Autodesk Inventor part; units mm, degrees
ref_plane "YZ Plane" through (0, 0, 0) normal (1, 0, 0) x (0, 1, 0)
ref_plane "XZ Plane" through (0, 0, 0) normal (0, 1, 0) x (-1, 0, 0)
ref_plane "XY Plane" through (0, 0, 0) normal (0, 0, 1) x (1, 0, 0)
sketch "スケッチ1" plane through (0, 0, 0) normal (1, 0, 0) x (0, 1, 0)
  line L0 (0, 0) -> (30, 0)
  line L1 (30, 0) -> (30, -43)
  line L2 (30, -43) -> (0, -43)
  line L3 (0, -43) -> (0, 0)
  circle A0 centre (15, -5) radius 1.5
  circle A1 centre (15, -38) radius 1.5
  line L4 (30, -21.5) -> (0, -21.5)
  line L5 (30, -18.3) -> (0, -18.3)
  line L6 (30, -24.7) -> (0, -24.7)
  line L7 (15, 0) -> (15, -43)
  line L8 (16.285, -18.3) -> (16.285, -24.7)
  line L9 (13.715, -18.3) -> (13.715, -24.7)
  line L10 (20.08, -18.3) -> (20.08, -24.7)
  line L11 (25.16, -18.3) -> (25.16, -24.7)
  line L12 (30.24, -18.3) -> (30.24, -24.7)
  line L13 (21.365, -18.3) -> (21.365, -24.7)
  line L14 (26.445, -18.3) -> (26.445, -24.7)
  line L15 (28.955, -18.3) -> (28.955, -24.7)
  line L16 (23.875, -18.3) -> (23.875, -24.7)
  line L17 (18.795, -18.3) -> (18.795, -24.7)
  line L18 (8.635, -18.3) -> (8.635, -24.7)
  line L19 (3.555, -18.3) -> (3.555, -24.7)
  line L20 (1.045, -18.3) -> (1.045, -24.7)
  line L21 (6.125, -18.3) -> (6.125, -24.7)
  line L22 (11.205, -18.3) -> (11.205, -24.7)
  circle A2 centre (5, -5) radius 1.6
  circle A3 centre (22.5, -5) radius 1.7
  circle A4 centre (22.5, -38) radius 1.7
  circle A5 centre (5, -38) radius 1.6
  line L23 (1.045, -18.3) -> (1.045, -24.7)
  line L24 (-1.525, -18.3) -> (-1.525, -24.7)
  line L25 (-4.035, -18.3) -> (-4.035, -24.7)
  line L26 (-6.605, -18.3) -> (-6.605, -24.7)
  line L27 (-6.605, -18.3) -> (-4.035, -18.3)
  line L28 (-5.32, -18.3) -> (-5.32, 0.2949)
  line L29 (-5.32, 0) -> (0, 0)
  line L30 (0, 0) -> (0, -43)
  line L31 (0, -43) -> (-5.32, -43)
  line L32 (-5.32, -43) -> (-5.32, 0)
  line L33 (0, -18.3) -> (-5.32, -18.3)
  line L34 (0, -24.7) -> (-5.32, -24.7)
  point P0 (15, -24.7)
  point P1 (15, -18.3)
  dimension "d0" = 30
  dimension "d1" = 43
  dimension "d2" = 3
  dimension "d3" = 3
  dimension "d4" = 5
  dimension "d5" = 5
  dimension "d6" = 15
  dimension "d7" = 15
  dimension "d8" = 3.2
  dimension "d9" = 3.2
  dimension "d10" = 1.285
  dimension "d11" = 1.285
  dimension "d12" = 5.08
  dimension "d13" = 5.08
  dimension "d14" = 5.08
  dimension "d15" = 1.285
  dimension "d16" = 1.285
  dimension "d17" = 1.285
  dimension "d21" = 3.2
  dimension "d22" = 3.4
  dimension "d23" = 3.4
  dimension "d24" = 3.2
  dimension "d25" = 5
  dimension "d26" = 5
  dimension "d28" = 7.5
  dimension "d30" = 5
  dimension "d31" = 7.5
  dimension "d32" = 5
  dimension "d38" = 5.08
  dimension "d43" = 0
  dimension "d44" = 10
  dimension "d45" = 10
extrude "押し出し1" add sketch "スケッチ1" along normal blind 4 contours L0 L7 A0 L5 L3 | L3 L33 L27 L28 L29 | L7 A0 | L5 L19 L4 L20 | L24 L34 L25 L33 | L6 L7 A1 L2 L3 | L3 L31 L32 L34 | L4 L19 L6 L20 | L7 L4 L9 L5 | L5 L18 L4 L21 | L9 L4 L22 L5 | L7 L6 L9 L4 | L4 L18 L6 L21 | L9 L6 L22 L4 | A1 L7 picked at (14.3164, -4.583) picked at (14.3492, -38.284)
sketch "スケッチ2" plane through (4, 0, 0) normal (1, 0, 0) x (0, 0, -1)
  line L0 (18.3, 1.045) -> (24.7, 1.045)
  line L1 (18.3, 3.555) -> (18.3, 6.125)
  line L2 (18.3, 6.125) -> (24.7, 6.125)
  line L3 (24.7, 6.125) -> (24.7, 3.555)
  line L4 (24.7, 3.555) -> (18.3, 3.555)
  line L5 (18.3, 11.205) -> (24.7, 11.205)
  line L6 (24.7, 11.205) -> (24.7, 8.635)
  line L7 (24.7, 8.635) -> (18.3, 8.635)
  line L8 (18.3, 8.635) -> (18.3, 11.205)
  line L9 (43, 15) -> (0, 15)
  line L10 (0, 15) -> (0, -5.32)
  line L11 (0, -5.32) -> (18.3, -5.32)
  line L12 (18.3, -5.32) -> (18.3, -4.035)
  line L13 (18.3, -4.035) -> (24.7, -4.035)
  line L14 (24.7, -4.035) -> (24.7, -5.32)
  line L15 (24.7, -5.32) -> (43, -5.32)
  line L16 (43, -5.32) -> (43, 15)
  line L17 (18.3, -1.525) -> (18.3, 1.045)
  line L18 (24.7, 1.045) -> (24.7, -1.525)
  line L19 (24.7, -1.525) -> (18.3, -1.525)
  point P0 (0, 0)
extrude "押し出し2" add sketch "スケッチ1" against normal blind 1 contours L0 L7 A0 L5 L3 | L3 L33 L27 L28 L29 | L7 A0 | L6 L7 A1 L2 L3 | L3 L31 L32 L34 | A1 L7 picked at (14.3164, -4.583) picked at (14.3492, -38.284)
fillet "フィレット3" radius 2 2 edges at (1.5, -5.32, 0) (1.5, -5.32, -43)
equation "\"d24\" = d21"
equation "\"d45\" = d44"
properties part number "RZvector-v1-Plate-B-F" material "ABS プラスチック"
Geometry: final body of the model. Coordinates: model frame, mm. A direction names the side the tool comes from. Coordinates: 2 decimals unless noted, no trailing zeros. Order: outer loops, then holes, each group sorted by start corner. A loop starts at its lowest first (then second) coordinate and runs counter-clockwise, first axis right, second up. Notation, with made-up numbers: M -5,-3.5 L 31,-3.5 A25 ccw 31,23.5 Z; hole C 7.5,35 d8. An arc over 180 degrees is marked long. Answer in a Markdown table with one row per item. Add a question column.
Q1. Section query B-B on x = 1.4. Return the cut outline in (y, z) (3 decimals).
Q2. Section query C-C on y = -0.5. Return the cut outline in (x, z), and give its area (3 significant figures).
Q3. Mould query, pull axis Y, two halves, no side actions, for faces 1 (the flat face through (1, 15, -21)), 2 (the flat face through (1, 6, -43)), 3 (the flat face through (2, 8.635, -21)). Classes: released by +Y, released by -Y, zero draft, split by the parting line, or undercut.
Q4. Reachability of faces 4 (the flat face through (2, 1.045, -21)), 5 (the flat face through (0, 13, -21)), 6 (the flat face through (2, -4.035, -21)), 7 (the flat face through (1, 5, -24.7)), 8 (the flat face through (-1, 5, -34)) from +Z, -Z, +X, -X, +Y, -Y: full face, straight path, thin tool, end or side. Return the list, or none.
Q5. Section query D-D on y = 5. Return the cut outline in (x, z).
Q6. Section query A-A on z = -5. Return the cut outline in (x, y), and give its area (3 significant figures).
Q7. Line query: L1, parallel to Z at x = 0.1, y = 5; L2, parallel to Y at x = 3.15, z = -22 (3 decimals); L3, parallel to X at y = 7.5, z = -21.5. Output: solid intervals per line, ascending.
Q8. Contact query for flat-ended pins moving along their axis: P1, Ø3, axis at x = 3, z = -21, coming from the -Y side (3 decimals); P2, Ø1.1, axis at y = 14, z = -21, coming from the -X side. Output: stop coordinate, or through.
Completed:
| question | item | result |
|---|---|---|
| 1 | outline | M -5.32,-41 A2 ccw -3.32,-43 L 15,-43 L 15,0 L -3.32,0 A2 ccw -5.32,-2 L -5.32,-18.3 L -4.035,-18.3 L -4.035,-24.7 L -5.32,-24.7 Z; hole M -1.525,-24.7 L 1.045,-24.7 L 1.045,-18.3 L -1.525,-18.3 Z; hole C 5,-38 d3.2; hole C 5,-5 d3.2; hole M 3.555,-24.7 L 6.125,-24.7 L 6.125,-18.3 L 3.555,-18.3 Z; hole M 8.635,-24.7 L 11.205,-24.7 L 11.205,-18.3 L 8.635,-18.3 Z |
| 2 | outline | M -1,-43 L 4,-43 L 4,-24.7 L -1,-24.7 Z; M -1,-18.3 L 4,-18.3 L 4,0 L -1,0 Z |
| 2 | area | 183 mm2 |
| 3 | face 1 | released by +Y |
| 3 | face 2 | zero draft |
| 3 | face 3 | undercut |
| 4 | face 4 | +X, -X |
| 4 | face 5 | -X, +Y, -Y |
| 4 | face 6 | +X, -X, -Y |
| 4 | face 7 | -X |
| 4 | face 8 | +Z, -Z, -X, +Y, -Y |
| 5 | outline | M -1,-43 L 4,-43 L 4,-39.6 L -1,-39.6 Z; M -1,-36.4 L 4,-36.4 L 4,-24.7 L -1,-24.7 Z; M -1,-18.3 L 4,-18.3 L 4,-6.6 L -1,-6.6 Z; M -1,-3.4 L 4,-3.4 L 4,0 L -1,0 Z |
| 6 | outline | M -1,-5.32 L 4,-5.32 L 4,3.4 L -1,3.4 Z; M -1,6.6 L 4,6.6 L 4,15 L -1,15 Z |
| 6 | area | 85.6 mm2 |
| 7 | L1 | z = -43 to -39.6, -36.4 to -24.7, -18.3 to -6.6, -3.4 to 0 |
| 7 | L2 | y = -4.035 to -1.525, 1.045 to 3.555, 6.125 to 8.635, 11.205 to 15 |
| 7 | L3 | x = 0 to 4 |
| 8 | P1 | stops at y = -4.035 |
| 8 | P2 | stops at x = 0 |
